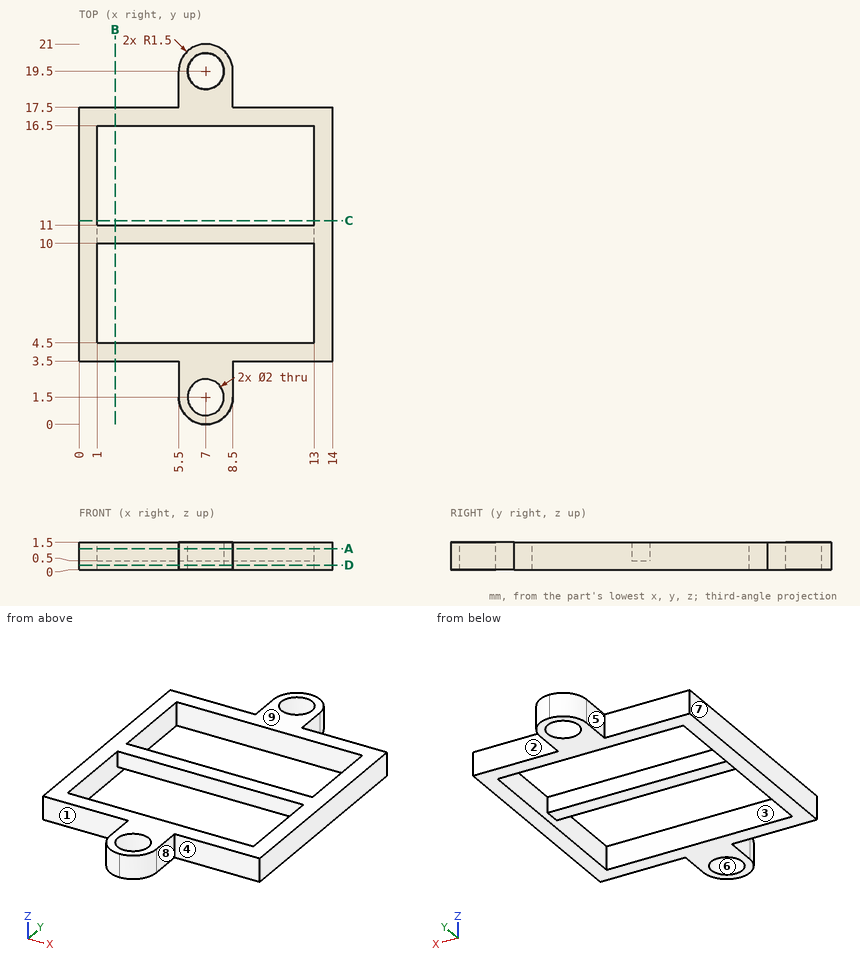
For this review, use the dimensioned drawing (mm, ordinates from the lowest corner) and the shaded views. A direction names the side the tool comes from. Give positions to 0.01 mm unless a question says otherwise; leave off trailing zeros. Loops run counter-clockwise (first coordinate to the right, second up) from the corner with the lowest first, then second, coordinate; pieces in that order, holes last. Notation, with made-up numbers: (-31, 80.5) -> (-24, 80.5) arc R36 ccw to (-24, 119.5) -> close; hole circle Ø7 at (34, 54). An arc over 180 degrees is marked (long way). Use CSV: the item, a comma, the result in double quotes.
1. For P1, Ø0.8, axis at x = 9.5, z = 1, coming from the +Y side, flat-tipped, find the tip position at first contact; note if it passes through.
Result:
P1,"stops at y = 17.5"
2. The part is to be moulded in two halves that separate along X. For the marked faces 6, 7, 8 and 9, say which applies: +X half, -X half, draft (parallel to the pull), parting line (faces both ways), or undercut.
Result:
face 6,"undercut"
face 7,"-X half"
face 8,"+X half"
face 9,"draft"
3. Consider section B-B, the plane x = 2. Write out the cut boundary in (y, z), then the cut area to 3 significant figures.
Result:
outline,"(3.5, 0) -> (4.5, 0) -> (4.5, 1.5) -> (3.5, 1.5) -> close; (10, 0.5) -> (11, 0.5) -> (11, 1.5) -> (10, 1.5) -> close; (16.5, 0) -> (17.5, 0) -> (17.5, 1.5) -> (16.5, 1.5) -> close"
area,"4.00 mm²"
4. Consider section C-C, the plane y = 11.25. Write out the cut boundary in (x, z).
Result:
outline,"(0, 0) -> (1, 0) -> (1, 1.5) -> (0, 1.5) -> close; (13, 0) -> (14, 0) -> (14, 1.5) -> (13, 1.5) -> close"
5. Consider section A-A, the plane z = 1.15. Write out the cut boundary in (x, y), then the cut area to 3 significant figures.
Result:
outline,"(0, 3.5) -> (5.5, 3.5) -> (5.5, 1.5) arc R1.5 ccw to (8.5, 1.5) -> (8.5, 3.5) -> (14, 3.5) -> (14, 17.5) -> (8.5, 17.5) -> (8.5, 19.5) arc R1.5 ccw to (5.5, 19.5) -> (5.5, 17.5) -> (0, 17.5) -> close; hole (1, 4.5) -> (13, 4.5) -> (13, 10) -> (1, 10) -> close; hole (1, 11) -> (13, 11) -> (13, 16.5) -> (1, 16.5) -> close; hole circle Ø2 at (7, 1.5); hole circle Ø2 at (7, 19.5)"
area,"76.8 mm²"
6. To check wall thickness, follow probe 1 along Y at (x, z) = (7, 0.75); probe 2 along Y at (x, z) = (4.75, 1); probe 3 along Y at (x, z) = (9.25, 0.1). State the ranges of each line that lie inside material, in increasing order. Write a range as from..to.
Result:
probe 1,"y = 0..0.5, 2.5..4.5, 10..11, 16.5..18.5, 20.5..21"
probe 2,"y = 3.5..4.5, 10..11, 16.5..17.5"
probe 3,"y = 3.5..4.5, 16.5..17.5"
7. Consider section D-D, the plane z = 0.25. Write out the cut boundary in (x, y).
Result:
outline,"(0, 3.5) -> (5.5, 3.5) -> (5.5, 1.5) arc R1.5 ccw to (8.5, 1.5) -> (8.5, 3.5) -> (14, 3.5) -> (14, 17.5) -> (8.5, 17.5) -> (8.5, 19.5) arc R1.5 ccw to (5.5, 19.5) -> (5.5, 17.5) -> (0, 17.5) -> close; hole (1, 4.5) -> (13, 4.5) -> (13, 16.5) -> (1, 16.5) -> close; hole circle Ø2 at (7, 1.5); hole circle Ø2 at (7, 19.5)"
8. Machinability: for the marked faces 1, 2, 3, 4 and 5, which of the approach directions +Z, -Z, +X, -X, +Y, -Y give a long, thin tool a straight path to every point of the face, cutting with its end or side? Answer none if there is none.
Result:
face 1,"+Z, -Z, -X, -Y"
face 2,"+Z, -Z, +X, +Y"
face 3,"+Z, -Z"
face 4,"+Z, -Z, +X, -Y"
face 5,"+Z, -Z, -X, +Y"
